Design review of the part built by this model. Coordinates are the model's own, in mm. A direction names the side the tool comes from. Coordinates: 2 decimals unless noted, no trailing zeros. Loops run counter-clockwise (first coordinate to the right, second up) from the corner with the lowest first, then second, coordinate; pieces in that order, holes last. Notation, with made-up numbers: M 79,72 L 115,72 A26 ccw 115,95 Z; hole C 26,-23 d6. An arc over 180 degrees is marked long. Write item = value, one per line. Start each with the question number.
```python
from build123d import *

# Parameters (mm, degrees)
F_1_2_20_TAPPED_HOLE1_D     = 11.50874
F_1_2_20_TAPPED_HOLE1_DEPTH = 29.21
F_1_2_20_TAPPED_HOLE1_TIP   = 3.45757432
FILLET1_R                   = 3.175


with BuildPart() as part:
    # Sketch1 → Revolve2 (revolve)
    with BuildSketch(Plane.XY):
        Polygon((-25.4, -2.966632853), (-25.4, 6.558367147), (-19.05, 6.558367147), (-19.05, 95.458367147), (0, 95.458367147), (0, 0), (0, -53.766632853), (-19.05, -53.766632853), (-19.05, -2.966632853), align=None)
    revolve(axis=Axis((0, 95.458367147, 0), (0, -1, 0)))

    # 1/2-20 Tapped Hole1
    with Locations(Plane.ZX.offset(95.458367147)):
        with Locations((0, 0)):
            Hole(F_1_2_20_TAPPED_HOLE1_D / 2, depth=F_1_2_20_TAPPED_HOLE1_DEPTH)
            with Locations((0, 0, -(F_1_2_20_TAPPED_HOLE1_DEPTH + F_1_2_20_TAPPED_HOLE1_TIP / 2))):  # 118° drill point
                Cone(0, F_1_2_20_TAPPED_HOLE1_D / 2, F_1_2_20_TAPPED_HOLE1_TIP, mode=Mode.SUBTRACT)

    # Fillet1
    fillet1_edges = [part.edges().sort_by_distance(p)[0] for p in [
        (19.05, 6.558367147, 0),
        (19.05, -2.966632853, 0),
    ]]
    fillet(fillet1_edges, radius=FILLET1_R)


solid = part.part
```
(1) Insertion check: pin 1 (1 mm diameter, centred on x = 1, z = 2.5, fed in from +Y); pin 2 (10 mm diameter, centred on x = -0.5, y = 10, fed in from -Z); pin 3 (1 mm diameter, centred on y = 36.5, z = 9, fed in from +X). Each pin has a flat end and moves straight along its axis. Give the tip position at first contact, or say it passes through.
(2) Mouldability with a two-part tool opening along Z and no side actions: class faces 4 (the cylindrical face through (15.12, -29.62, 11.59)), 5 (the flat face through (0.1, 6.558, 22.5)), 6 (the conical face through (-0.976, 63.391, -0.217)) as +Z half, -Z half, draft (parallel to the pull), parting line (faces both ways), or undercut.
(3) Tool access review of faces 1 (the cylindrical face through (5.705, 80.649, 0.749)), 2 (the flat face through (-4, 95.458, -5)), 3 (the flat face through (-0.1, -2.967, 22.5)): name each direction out of +Z, -Z, +X, -X, +Y, -Y from which nothing blocks a thin tool from reaching the whole face with its end or side.
(4) Take a section at B-B (y = 69). State the section outline as (x, z) points, plus the area to 3 significant figures.
(5) To check wall thickness, follow L1, parallel to Z at x = 0, y = 77.5; L2, parallel to Y at x = -13.5, z = -17.5. State the ranges of each line that lie inside material, in increasing order.
(6) Take a section at A-A (y = 41). State the section outline as (x, z) points.
Results list:
q1.pin_1 = 64.71
q1.pin_2 = -25.4
q1.pin_3 = 17.05
q2.face_4 = parting line
q2.face_5 = draft
q2.face_6 = undercut
q3.face_1 = +Y
q3.face_2 = +Z, -Z, +X, -X, +Y
q3.face_3 = -Y
q4.outline = C 0,0 d38.1; hole C 0,0 d11.51
q4.area = 1,040 mm^2
q5.L1 = -19.05 to -5.75, 5.75 to 19.05
q5.L2 = -2.97 to 6.56
q6.outline = C 0,0 d38.1
